Work out the finished part from the listing and answer in its coordinate system (mm). A direction names the side the tool comes from. Coordinates: 2 decimals unless noted, no trailing zeros. Write each loop counter-clockwise with the first axis right and the second up, starting at its lowest first coordinate (ties: lowest second). Pieces come first, ordered by that corner, then holes. Notation, with made-up numbers: (72.25, 12) - (116.25, 12) arc R22 ccw to (116.25, 20) - close; hole circle Ø5 at (0, 72). An arc over 180 degrees is marked (long way). Use CSV: the item, a comma, the result in double quotes. Start each with the question number.
from build123d import *

# Parameters (mm, degrees)
SKETCH1_R           = 4
SKETCH1_R_2         = 1.5
BOSS_EXTRUDE1_DEPTH = 15
BOSS_EXTRUDE2_START = -5
SKETCH2_R           = 1.5
BOSS_EXTRUDE2_DEPTH = 5
SKETCH3_R           = 2.5
BOSS_EXTRUDE3_DEPTH = 60


with BuildPart() as part:
    # Sketch1 → Boss-Extrude1 (new body)
    with BuildSketch(Plane.XY):
        Circle(SKETCH1_R)
        Circle(SKETCH1_R_2, mode=Mode.SUBTRACT)
    extrude(amount=BOSS_EXTRUDE1_DEPTH)

    # Sketch2 → Boss-Extrude2 (add)
    with BuildSketch(Plane.XY.offset(15).offset(BOSS_EXTRUDE2_START)):
        Circle(SKETCH2_R)
    extrude(amount=BOSS_EXTRUDE2_DEPTH)

    # Sketch3 → Boss-Extrude3 (add)
    with BuildSketch(Plane.XY.offset(15)):
        Circle(SKETCH3_R)
    extrude(amount=BOSS_EXTRUDE3_DEPTH)


solid = part.part
Item 1: Straight lines are drawn through the part: probe 1 along Y at (x, z) = (0, 3); probe 2 along Z at (x, y) = (3, -2); probe 3 along Y at (x, z) = (2, 53). For each, find the intervals that lie inside material, in ascending order. Write a range as [from, to].
Item 2: Each of these flat-tipped pins is pushed along its axis until it touches: pin 1 (2 mm diameter, centred on y = -2, z = 11.5, fed in from +X); pin 2 (4 mm diameter, centred on x = 2.5, z = 21, fed in from -Y); pin 3 (2.5 mm diameter, centred on x = 0, y = 0, fed in from -Z). Where does it stop, or does it pass through?
Item 3: A cutting plane is placed at A-A (y = 0). Determine the outline of the cut face in (x, z), then the cut area to 3 significant figures.
Item 4: Which of the six approach directions +Z, -Z, +X, -X, +Y, -Y give full straight-line access (tool end or side, diameter ignored) to faces 1 (the face through (-0.54, -2.44, 44.58)), 2 (the face through (0, 0, 10)), 3 (the face through (2, 0, 0))?
Item 5: A cutting plane is placed at C-C (z = 34.5). Determine the outline of the cut face in (x, y).
Item 6: Determine the mould class of faces 4 (the face through (2, 2, 15)), 5 (the face through (-1.5, 0.07, 4.93)), 6 (the face through (-0.867, -3.905, 7.395)) for opening direction X: +X half, -X half, draft (parallel to the pull), parting line (faces both ways), or undercut.
Calculated:
1,probe 1,"y = [-4, -1.5], [1.5, 4]"
1,probe 2,"z = [0, 15]"
1,probe 3,"y = [-1.5, 1.5]"
2,pin 1,"stops at x = 3.87"
2,pin 2,"stops at y = -2.45"
2,pin 3,"stops at z = 10"
3,outline,"(-4, 0) - (-1.5, 0) - (-1.5, 10) - (1.5, 10) - (1.5, 0) - (4, 0) - (4, 15) - (2.5, 15) - (2.5, 75) - (-2.5, 75) - (-2.5, 15) - (-4, 15) - close"
3,area,"390 mm²"
4,face 1,"+Z"
4,face 2,"-Z"
4,face 3,"-Z, +X, -X, +Y, -Y"
5,outline,"circle Ø5 at (0, 0)"
6,face 4,"draft"
6,face 5,"undercut"
6,face 6,"parting line"
